Here's how the part is built. I have some questions about the finished solid (model axes, mm). A direction names the side the tool comes from. Round coordinates to 2 decimals unless told otherwise and drop trailing zeros. Order: outer loops, then holes, each group sorted by start corner. A loop starts at its lowest first (then second) coordinate and runs counter-clockwise, first axis right, second up. Notation, with made-up numbers: (12.5, 79.5) - (24.5, 79.5) arc R25 ccw to (24.5, 94.5) - close; hole circle Ø10 at (86.5, -14.5). An arc over 180 degrees is marked (long way). Answer as a JSON object with one key per item and string values.
```python
from build123d import *

# Parameters (mm, degrees)
BOSS_EXTRUDE1_DEPTH = 5.9944
CUT_EXTRUDE2_DEPTH  = 5.9944
SKETCH3_R           = 5.55625
CUT_EXTRUDE3_DEPTH  = 5.9944


with BuildPart() as part:
    # Sketch1 → Boss-Extrude1 (new body)
    with BuildSketch(Plane.XY):
        Polygon((25.4, 5.9944), (50.8, 5.9944), (50.8, 0), (76.2, 0), (76.2, 5.9944), (101.6, 5.9944), (101.6, 0), (127, 0), (127, 75.4888), (101.6, 75.4888), (101.6, 69.4944), (76.2, 69.4944), (76.2, 75.4888), (50.8, 75.4888), (50.8, 69.4944), (25.4, 69.4944), (25.4, 75.4888), (0, 75.4888), (0, 0), (25.4, 0), align=None)
    extrude(amount=BOSS_EXTRUDE1_DEPTH)

    # Sketch2 → Cut-Extrude2 (cut)
    with BuildSketch(Plane.XY.offset(5.9944)):
        Polygon((36.449, 69.4944), (36.449, 64.4144), (34.163, 64.4144), (34.163, 61.8744), (36.449, 61.8744), (36.449, 58.0644), (39.751, 58.0644), (39.751, 61.8744), (42.037, 61.8744), (42.037, 64.4144), (39.751, 64.4144), (39.751, 69.4944), align=None)
        Polygon((36.449, 5.9944), (39.751, 5.9944), (39.751, 11.0744), (42.037, 11.0744), (42.037, 13.6144), (39.751, 13.6144), (39.751, 17.4244), (36.449, 17.4244), (36.449, 13.6144), (34.163, 13.6144), (34.163, 11.0744), (36.449, 11.0744), align=None)
        Polygon((90.551, 5.9944), (90.551, 11.0744), (92.837, 11.0744), (92.837, 13.6144), (90.551, 13.6144), (90.551, 17.4244), (87.249, 17.4244), (87.249, 13.6144), (84.963, 13.6144), (84.963, 11.0744), (87.249, 11.0744), (87.249, 5.9944), align=None)
        Polygon((90.551, 69.4944), (87.249, 69.4944), (87.249, 64.4144), (84.963, 64.4144), (84.963, 61.8744), (87.249, 61.8744), (87.249, 58.0644), (90.551, 58.0644), (90.551, 61.8744), (92.837, 61.8744), (92.837, 64.4144), (90.551, 64.4144), align=None)
    extrude(amount=-CUT_EXTRUDE2_DEPTH, mode=Mode.SUBTRACT)

    # Sketch3 → Cut-Extrude3 (cut)
    with BuildSketch(Plane.XY.offset(5.9944)):
        with Locations((63.5, 37.7444)):
            Circle(SKETCH3_R)
    extrude(amount=-CUT_EXTRUDE3_DEPTH, mode=Mode.SUBTRACT)


solid = part.part
```
1. For faces 4 (the face through (84.963, 63, 3)), 5 (the face through (76.2, 72, 3)), 6 (the face through (82, 5.994, 3)), which set-ups out of +Z, -Z, +X, -X, +Y, -Y let a thin tool reach every point of the face, with its end or its side?
Responses:
{"face 4": "+Z, -Z", "face 5": "+Z, -Z, +Y", "face 6": "+Z, -Z, -Y"}
2. Imagine slicing it at C-C (x = 29). List the corners of the cut face in (y, z) for me.
Responses:
{"outline": "(5.99, 0) - (69.49, 0) - (69.49, 5.99) - (5.99, 5.99) - close"}
3. If I drill on L1, parallel to X at y = 66.5, z = 3.15; L2, parallel to X at y = 70.5, z = 5; L3, parallel to X at y = 38, z = 3.35, over which ranges is the centre line in solid material (lowest first)? Write a range as [from, to].
Responses:
{"L1": "[0, 36.45], [39.75, 87.25], [90.55, 127]", "L2": "[0, 25.4], [50.8, 76.2], [101.6, 127]", "L3": "[0, 57.95], [69.05, 127]"}
4. For P1, Ø1.3, axis at y = 63, z = 2.5, coming from the -X side; P2, Ø1.1, axis at x = 36, z = 4.5, coming from the +Y side; P3, Ø2.5, axis at x = 92, z = 1.5, coming from the -Y side, each with a flat end and sliding along its axis, tell me the tip position at first contact or that it passes through.
Responses:
{"P1": "x = 0", "P2": "y = 69.49", "P3": "y = 5.99"}
5. Imagine slicing it at B-B (y = 40). List the corners of the cut face in (x, z) for me.
Responses:
{"outline": "(0, 0) - (58.42, 0) - (58.42, 5.99) - (0, 5.99) - close; (68.58, 0) - (127, 0) - (127, 5.99) - (68.58, 5.99) - close"}
6. Imagine slicing it at A-A (x = 63.5). List the corners of the cut face in (y, z) for me, plus the area to 3 significant figures.
Responses:
{"outline": "(0, 0) - (32.19, 0) - (32.19, 5.99) - (0, 5.99) - close; (43.3, 0) - (75.49, 0) - (75.49, 5.99) - (43.3, 5.99) - close", "area": "386 mm2"}
7. Thinking about a two-plate mould opening in X: for faces 1 (the face through (45, 69.494, 3)), 2 (the face through (13, 75.489, 3)), 3 (the face through (127, 37, 3)), which applies, pulls with the +X half, pulls with the -X half, needs draft (parallel to the pull), parting line crosses it, or undercut?
Responses:
{"face 1": "undercut", "face 2": "needs draft", "face 3": "pulls with the +X half"}
